The model under review builds one solid part; all positions refer to its coordinate system, in mm. A direction names the side the tool comes from. Round coordinates to 2 decimals unless told otherwise and drop trailing zeros. Order: outer loops, then holes, each group sorted by start corner. A loop starts at its lowest first (then second) coordinate and runs counter-clockwise, first axis right, second up.
```python
from build123d import *
from OCP.BRepFilletAPI import BRepFilletAPI_MakeChamfer

# Parameters (mm, degrees)
SKETCH1_R               = 9.5
BOSS_EXTRUDE1_DEPTH     = 10
SKETCH6_R               = 6
BOSS_EXTRUDE2_DEPTH     = 10
SKETCH2_R               = 2.6
CUT_EXTRUDE1_DEPTH      = 10
SKETCH3_R               = 2.15
CUT_EXTRUDE2_DEPTH      = 17.748134224
CUT_EXTRUDE3_DEPTH      = 3.3
CUT_EXTRUDE4_DEPTH      = 2.7
CUT_EXTRUDE5_REACH      = 25.479
CUT_EXTRUDE5_END_RADIUS = 2.6
SKETCH7_R               = 1.65
FILLET1_R               = 3
CHAMFER1_SIZE           = 0.356629571
CHAMFER1_SIZE_2         = 0.5
CHAMFER2_SIZE           = 0.5
FILLET2_R               = 1.5


with BuildPart() as part:
    # Sketch1 → Boss-Extrude1 (new body)
    with BuildSketch(Plane.XY):
        Circle(SKETCH1_R)
    extrude(amount=BOSS_EXTRUDE1_DEPTH)

    # Sketch6 → Boss-Extrude2 (add)
    with BuildSketch(Plane(origin=(0, 0, 0), x_dir=(-1, 0, 0), z_dir=(0, 0, -1))):
        with Locations(Location((0, 0, 0), (0, 0, 180))):
            Circle(SKETCH6_R)
    extrude(amount=BOSS_EXTRUDE2_DEPTH)

    # Sketch2 → Cut-Extrude1 (cut)
    with BuildSketch(Plane.XY.offset(10)):
        Circle(SKETCH2_R)
    extrude(amount=-CUT_EXTRUDE1_DEPTH, mode=Mode.SUBTRACT)

    # Sketch3 → Cut-Extrude2 (cut, through all)
    with BuildSketch(Plane.XY):
        Circle(SKETCH3_R)
    extrude(amount=-CUT_EXTRUDE2_DEPTH, mode=Mode.SUBTRACT)

    # Sketch4 → Cut-Extrude3 (cut)
    with BuildSketch(Plane(origin=(0, 0, -7), x_dir=(-1, 0, 0), z_dir=(0, 0, -1))):
        Polygon((-3.65, -9.105308986), (3.65, -9.105308986), (3.65, 2.107328483), (0, 4.214656965), (-3.65, 2.107328483), align=None)
    extrude(amount=-CUT_EXTRUDE3_DEPTH, mode=Mode.SUBTRACT)

    # Sketch5 → Cut-Extrude4 (cut)
    with BuildSketch(Plane(origin=(0, 4, 0), x_dir=(-1, 0, 0), z_dir=(0, 1, 0))):
        Polygon((-2.85, 11.49401058), (2.85, 11.49401058), (2.85, 4.354551733), (0, 2.709103466), (-2.85, 4.354551733), align=None)
    extrude(amount=CUT_EXTRUDE4_DEPTH, mode=Mode.SUBTRACT)

    # Cut-Extrude5: up to this cylinder (the profile starts outside it)
    cut_extrude5_end = Plane(origin=(0, 0, 5.88453), z_dir=(0, 0, 1)) * Cylinder(CUT_EXTRUDE5_END_RADIUS, 57.158, mode=Mode.PRIVATE)
    # Sketch7 → Cut-Extrude5 (cut, up to the surface)
    with BuildSketch(Plane(origin=(0, 9.5, 0), x_dir=(-1, 0, 0), z_dir=(0, 1, 0)), mode=Mode.PRIVATE) as cut_extrude5_sk1:
        with Locations(Location((0, 5.884529946, 0), (0, 0, 90))):
            Circle(SKETCH7_R)
    cut_extrude5_tool1 = extrude(cut_extrude5_sk1.sketch, amount=-CUT_EXTRUDE5_REACH, mode=Mode.PRIVATE) - cut_extrude5_end
    add(cut_extrude5_tool1.solids().sort_by_distance((0, 9.5, 5.88453))[0], mode=Mode.SUBTRACT)

    # Fillet1
    fillet1_edges = [part.edges().sort_by_distance(p)[0] for p in [
        (-6, 0, 0),
    ]]
    fillet(fillet1_edges, radius=FILLET1_R)

    # Chamfer1
    chamfer1_edges_1 = [part.edges().sort_by_distance(p)[0] for p in [
        (-3.65, -4.762089877, -5.35),
    ]]
    chamfer1_side_1 = [part.faces().sort_by_distance(p)[0] for p in [
        (-3.655661007, -4.757750884, -5.35),
    ]]
    chamfer1_edges_2 = [part.edges().sort_by_distance(p)[0] for p in [
        (3.65, -4.762089877, -5.35),
    ]]
    chamfer1_side_2 = [part.faces().sort_by_distance(p)[0] for p in [
        (3.655661007, -4.757750884, -5.35),
    ]]
    chamfer1 = BRepFilletAPI_MakeChamfer(part.part.solid().wrapped)
    for e in chamfer1_edges_1:
        chamfer1.Add(CHAMFER1_SIZE - 0.0004, CHAMFER1_SIZE_2 - 0.0004, e.wrapped, chamfer1_side_1[0].wrapped)
    for e in chamfer1_edges_2:
        chamfer1.Add(CHAMFER1_SIZE - 0.0004, CHAMFER1_SIZE_2 - 0.0004, e.wrapped, chamfer1_side_2[0].wrapped)
    add(Compound.cast(chamfer1.Shape()), mode=Mode.REPLACE)  # a hair under: the kernel refuses the full size

    # Chamfer2
    chamfer2_edges = [part.edges().sort_by_distance(p)[0] for p in [
        (-2.85, 5.35, 10),
        (2.85, 5.35, 10),
    ]]
    chamfer(chamfer2_edges, length=CHAMFER2_SIZE)

    # Fillet2
    fillet2_edges = [part.edges().sort_by_distance(p)[0] for p in [
        (-9.5, 0, 10),
    ]]
    fillet(fillet2_edges, radius=FILLET2_R)


solid = part.part
```
(1) Consider section A-A (y = 0). Write out the cut boundary in (x, z).
Data:
outline: (-9.5, 0) - (-9, 0) arc R3 cw to (-6, -3) - (-6, -10) - (-2.15, -10) - (-2.15, -7) - (-3.65, -7) - (-3.65, -3.7) - (-2.15, -3.7) - (-2.15, 0) - (-2.6, 0) - (-2.6, 10) - (-8, 10) arc R1.5 ccw to (-9.5, 8.5) - close; (2.15, -10) - (6, -10) - (6, -3) arc R3 cw to (9, 0) - (9.5, 0) - (9.5, 8.5) arc R1.5 ccw to (8, 10) - (2.6, 10) - (2.6, 0) - (2.15, 0) - (2.15, -3.7) - (3.65, -3.7) - (3.65, -7) - (2.15, -7) - close
(2) Draft analysis for pull direction Z (two halves, no side actions). For faces 1 (the flat face through (-1.44, 5.33, 3.54)), 2 (the flat face through (0, 4, 8)), 3 (the flat face through (1.799, 3.176, -5.373)), state which applies: pulls with the +Z half, pulls with the -Z half, needs draft (parallel to the pull), parting line crosses it, or undercut.
Data:
face 1: pulls with the +Z half
face 2: needs draft
face 3: undercut
(3) To check wall thickness, follow probe 1 along Y at (x, z) = (0, 3.25); probe 2 along Z at (x, y) = (-3.5, -3.75); probe 3 along Y at (x, z) = (0, -8.65). State the ranges of each line that lie inside material, in increasing order.
Data:
probe 1: y = -9.5 to -2.6, 2.6 to 4, 6.7 to 9.5
probe 2: z = -10 to -7, -3.7 to 10
probe 3: y = -6 to -2.15, 2.15 to 6
(4) Consider section D-D (y = 3.25). State how many separate pieces and enclosed holes the cut face has, and give its area (3 significant figures).
Data:
separate pieces: 1
enclosed holes: 2
area: 263 mm2
(5) Consider section B-B (z = -6). Write out the cut boundary in (x, y), and give its area (3 significant figures).
Data:
outline: (-3.93, -4.54) - (-3.65, -4.26) - (-3.65, 2.11) - (0, 4.21) - (3.65, 2.11) - (3.65, -4.26) - (3.93, -4.54) arc R6 ccw (long way) to start
area: 49.0 mm2
(6) Insertion check: pin 1 (2 mm diameter, centred on y = 6, z = 5.5, fed in from -X); pin 2 (1.6 mm diameter, centred on y = -1.5, z = -6, fed in from +X); pin 3 (10 mm diameter, centred on x = 6, z = -2, fed in from +Y); pin 4 (4 mm diameter, centred on x = 0, y = 0, fed in from +Z). Each pin has a flat end and moves straight along its axis. Give the tip position at first contact, or say it passes through.
Data:
pin 1: stops at x = -8.08
pin 2: stops at x = 5.96
pin 3: stops at y = 9.39
pin 4: passes through
(7) For faces 4 (the cylindrical face through (1.39, 3.24, 6.77)), 5 (the flat face through (0, 6.7, 8)), 6 (the flat face through (-1.851, 3.146, -5.373)), list the 3-axis set-ups (+Z, -Z, +X, -X, +Y, -Y) from which the entire face can be reached by the end or side of a thin tool; tool diameter is ignored.
Data:
face 4: +Y
face 5: +Z
face 6: -Y
(8) Consider section C-C (z = -2). Write out the cut boundary in (x, y), and give its area (3 significant figures).
Data:
outline: circle Ø12.34 at (0, 0); hole circle Ø4.3 at (0, 0)
area: 105 mm2
